Can you work these out from the model? Positions are in its coordinate system, mm. Face numbers are marked on the shaded views. A direction names the side the tool comes from. Round coordinates to 2 decimals unless told otherwise and drop trailing zeros. Order: outer loops, then holes, each group sorted by start corner. A loop starts at its lowest first (then second) coordinate and runs counter-clockwise, first axis right, second up. Notation, with made-up numbers: (73, 83.25) - (100, 83.25) arc R19 cw to (100, 104.25) - close; hole circle Ø1 at (-3, 14.25). An arc over 180 degrees is marked (long way). Write item = value, one per line.
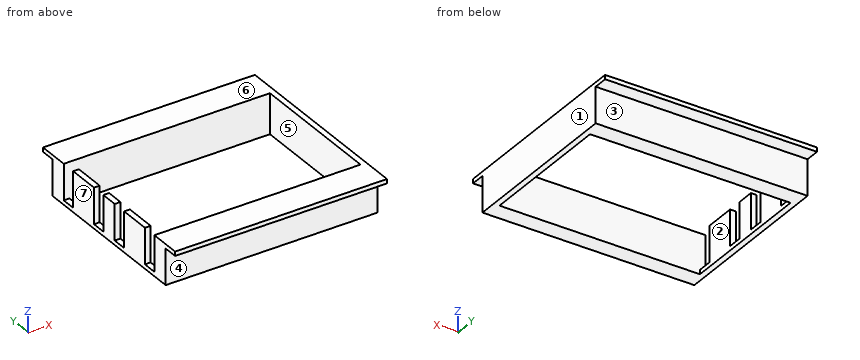
Autodesk Inventor part; units mm, degrees
ref_plane "YZ Plane" through (0, 0, 0) normal (1, 0, 0) x (0, 1, 0)
ref_plane "XZ Plane" through (0, 0, 0) normal (0, 1, 0) x (-1, 0, 0)
ref_plane "XY Plane" through (0, 0, 0) normal (0, 0, 1) x (1, 0, 0)
sketch "Esquisse1" plane through (0, 0, 0) normal (0, 0, 1) x (1, 0, 0)
  line L0 (-70, 48) -> (70, 48)
  line L1 (70, 48) -> (70, -48)
  line L2 (70, -48) -> (-70, -48)
  line L3 (-70, -48) -> (-70, 48)
  line L4 (74, -60) -> (-74, -60)
  line L5 (-74, -60) -> (-74, 60)
  line L6 (-74, 60) -> (74, 60)
  line L7 (74, 60) -> (74, -60)
  line L8 (74, -60) -> (-74, 60) construction
  line L9 (-74, -60) -> (74, 60) construction
  point P0 (0, 0)
  dimension "d0" = 48
  dimension "d1" = 48
  dimension "d2" = 70
  dimension "d3" = 70
  dimension "d4" = 60
  dimension "d5" = 74
extrude "Extrusion1" add sketch "Esquisse1" along normal blind 28
sketch "Esquisse3" plane through (-74, -60, 28) normal (-1, 0, 0) x (0, 0, 1)
  line L0 (-28, 108) -> (0, 108)
  line L1 (-28, 48) -> (-28, 4)
  line L2 (0, 108) -> (-28, 108)
  line L3 (-28, 108) -> (-28, 98)
  line L4 (-28, 98) -> (0, 98)
  line L5 (0, 98) -> (0, 108)
  line L6 (-28, 12) -> (0, 12)
  line L7 (0, 12) -> (-28, 12)
  line L8 (-28, 12) -> (-28, 22)
  line L9 (-28, 22) -> (0, 22)
  line L10 (0, 22) -> (0, 12)
  line L11 (-28, 12) -> (-28, 108)
  line L12 (0, 12) -> (0, 108)
  line L13 (-28, 44) -> (0, 44)
  line L14 (0, 44) -> (0, 54)
  line L15 (0, 54) -> (-28, 54)
  line L16 (-28, 54) -> (-28, 44)
  line L17 (-28, 66) -> (0, 66)
  line L18 (0, 66) -> (0, 76)
  line L19 (0, 76) -> (-28, 76)
  line L20 (-28, 76) -> (-28, 66)
  point P0 (-28, 60)
  point P1 (0, 12)
  point P2 (-28, 22)
  point P3 (0, 66)
  point P4 (0, 44)
  dimension "d10" = 10
  dimension "d11" = 10
  dimension "d12" = 28
  dimension "d13" = 28
  dimension "d29" = 42
  dimension "d30" = 42
  dimension "d31" = 10
  dimension "d32" = 10
extrude "Extrusion3" cut sketch "Esquisse3" against normal blind 10 contours L0 L5 L4 L3 | L19 L12 L17 L11 | L15 L12 L13 L1 L11 | L10 L6 L1 L9
sketch "Esquisse4" plane through (-74, 60, 28) normal (0, 1, 0) x (1, 0, 0)
  line L0 (148, 28) -> (148, 0)
  line L1 (144, 0) -> (4, 0)
  line L2 (148, 3) -> (0, 3)
  line L3 (0, 3) -> (0, 0)
  line L4 (0, 0) -> (148, 0)
  line L5 (148, 0) -> (148, 3)
  point P0 (74, 28)
  point P1 (148, 31)
  point P2 (148, 0)
  dimension "d21" = 3
extrude "Extrusion4" add sketch "Esquisse4" along normal blind 10
sketch "Esquisse5" plane through (-74, -60, 28) normal (0, -1, 0) x (1, 0, 0)
  line L0 (0, 0) -> (144, 0)
  line L1 (148, -28) -> (148, -3)
  line L2 (0, 0) -> (148, 0)
  line L3 (148, 0) -> (148, -3)
  line L4 (148, -3) -> (0, -3)
  line L5 (0, -3) -> (0, 0)
  point P0 (74, -28)
  point P1 (148, -31)
  point P2 (4, 0)
  point P3 (4, 0)
  dimension "d22" = 3
extrude "Extrusion5" add sketch "Esquisse5" along normal blind 10
sketch "Esquisse6" plane through (-74, -38, 0) normal (-1, 0, 0) x (0, 0, 1)
  line L0 (0, 86) -> (28, 86)
  line L1 (0, -10) -> (28, -10)
  line L2 (0, -10) -> (0, -22)
  line L3 (0, -10) -> (3, -10)
  line L4 (3, -10) -> (3, 86)
  line L5 (3, 86) -> (0, 86)
  line L6 (0, 86) -> (0, -10)
  point P0 (0, 38)
  dimension "d28" = 3
extrude "Extrusion6" add sketch "Esquisse6" against normal blind 4
properties part number "Support_batterie"
(1) Will these pins go through, and if not, where does the flat tip stop? P1, Ø2, axis at x = -73, z = 17, coming from the +Y side; P2, Ø2, axis at x = -72.5, y = 9, coming from the +Z side; P3, Ø3, axis at x = 13.5, y = -65, coming from the -Z side.
Computed:
P1 = 60
P2 = 3
P3 = 25
(2) If we section it at A-A (z = 6.75): Write out the boundary of the cut face in (x, y).
Computed:
outline = (-74, -60) - (74, -60) - (74, 60) - (-74, 60) - (-74, 48) - (70, 48) - (70, -48) - (-74, -48) - close; (-74, -38) - (-70, -38) - (-70, -16) - (-74, -16) - close; (-74, -6) - (-70, -6) - (-70, 6) - (-74, 6) - close; (-74, 16) - (-70, 16) - (-70, 38) - (-74, 38) - close
(3) If we section it at C-C (y = -20.5): Write out the boundary of the cut face in (x, z).
Computed:
outline = (-74, 0) - (-70, 0) - (-70, 28) - (-74, 28) - close; (70, 0) - (74, 0) - (74, 28) - (70, 28) - close
(4) If we section it at B-B (x = -32): Write out the boundary of the cut face in (y, z).
Computed:
outline = (-70, 25) - (-60, 25) - (-60, 0) - (-48, 0) - (-48, 28) - (-70, 28) - close; (48, 0) - (60, 0) - (60, 25) - (70, 25) - (70, 28) - (48, 28) - close
(5) On a 3-axis mill with a long thin cutter (end or side, diameter ignored), from which of +Z, -Z, +X, -X, +Y, -Y can I reach the whole of each face in a straight line? I mean the marked faces 1, 2, 3 and 4. Say none if no direction works.
Computed:
face_1 = +Z, -Z, +X, +Y, -Y
face_2 = +Z, -Z
face_3 = -Z, +X, -X, +Y
face_4 = -Z, +X, -X, -Y
(6) Thinking about a two-plate mould opening in X: for the marked faces 5, 6 and 7, which applies, +X half, -X half, draft (parallel to the pull), parting line (faces both ways), or undercut?
Computed:
face_5 = undercut
face_6 = draft
face_7 = -X half
(7) If I drill on line 1 (X direction, y = -16.5, z = 7); line 2 (Y direction, x = -2, z = 26); line 3 (Y direction, x = -32.5, z = 4.25), over which ranges is the centre line in solid material (lowest first)? Write a range as from..to.
Computed:
line_1 = -74..-70, 70..74
line_2 = -70..-48, 48..70
line_3 = -60..-48, 48..60
